Check sheet for the modelled part. Datum: model origin and axes. Units: mm. A direction names the side the tool comes from. Round coordinates to 2 decimals unless told otherwise and drop trailing zeros. Write each loop counter-clockwise with the first axis right and the second up, starting at its lowest first coordinate (ties: lowest second). Pieces come first, ordered by that corner, then holes. Notation, with made-up numbers: M 8.25,2.25 L 16.25,2.25 A19 ccw 16.25,11.25 Z; hole C 77.5,-1.5 d1. An arc over 180 degrees is marked long. Answer in a Markdown table with one row per item.
```python
from build123d import *

# Parameters (mm, degrees)
F1_DEPTH = 3.81


with BuildPart() as f1:
    # F0 (on Front) → F1 (new body)
    with BuildSketch(Plane.XZ):
        Polygon((24.534516, 6.574004), (0, 0), (25.4, 0), (19.930718, 2.623929), align=None)
        Polygon((-6.574004, 24.534516), (0, 0), (0, 25.4), (-2.623929, 19.930718), align=None)
        Polygon((-24.534516, -6.574004), (0, 0), (-25.4, 0), (-19.930718, -2.623929), align=None)
        Polygon((6.574004, -24.534516), (0, 0), (0, -25.4), (2.623929, -19.930718), align=None)
        Polygon((25.4, 0), (0, 0), (24.534516, -6.574004), (19.930718, -2.623929), align=None)
        Polygon((21.997045, 12.7), (0, 0), (24.534516, 6.574004), (18.572473, 7.69297), align=None)
        Polygon((17.960512, 17.960512), (0, 0), (21.997045, 12.7), (15.948544, 12.237748), align=None)
        Polygon((12.7, 21.997045), (0, 0), (17.960512, 17.960512), (12.237748, 15.948544), align=None)
        Polygon((6.574004, 24.534516), (0, 0), (12.7, 21.997045), (7.69297, 18.572473), align=None)
        Polygon((0, 25.4), (0, 0), (6.574004, 24.534516), (2.623929, 19.930718), align=None)
        Polygon((0, -25.4), (0, 0), (-6.574004, -24.534516), (-2.623929, -19.930718), align=None)
        Polygon((24.534516, -6.574004), (0, 0), (21.997045, -12.7), (18.572473, -7.69297), align=None)
        Polygon((21.997045, -12.7), (0, 0), (17.960512, -17.960512), (15.948544, -12.237748), align=None)
        Polygon((17.960512, -17.960512), (0, 0), (12.7, -21.997045), (12.237748, -15.948544), align=None)
        Polygon((12.7, -21.997045), (0, 0), (6.574004, -24.534516), (7.69297, -18.572473), align=None)
        Polygon((-6.574004, -24.534516), (0, 0), (-12.7, -21.997045), (-7.69297, -18.572473), align=None)
        Polygon((-12.7, -21.997045), (0, 0), (-17.960512, -17.960512), (-12.237748, -15.948544), align=None)
        Polygon((-17.960512, -17.960512), (0, 0), (-21.997045, -12.7), (-15.948544, -12.237748), align=None)
        Polygon((-21.997045, -12.7), (0, 0), (-24.534516, -6.574004), (-18.572473, -7.69297), align=None)
        Polygon((-25.4, 0), (0, 0), (-24.534516, 6.574004), (-19.930718, 2.623929), align=None)
        Polygon((-24.534516, 6.574004), (0, 0), (-21.997045, 12.7), (-18.572473, 7.69297), align=None)
        Polygon((-21.997045, 12.7), (0, 0), (-17.960512, 17.960512), (-15.948544, 12.237748), align=None)
        Polygon((-17.960512, 17.960512), (0, 0), (-12.7, 21.997045), (-12.237748, 15.948544), align=None)
        Polygon((-12.7, 21.997045), (0, 0), (-6.574004, 24.534516), (-7.69297, 18.572473), align=None)
    extrude(amount=F1_DEPTH)


solid = f1.part
```
1. Section check A-A, the plane z = -5. Record the cut outline in (x, y).
Found:
| item | result |
|---|---|
| outline | M -22.7,-3.81 L 22.7,-3.81 L 22.7,0 L -22.7,0 Z |
2. Draft check along Z on faces 5 (the face through (10.16, -1.88, -20.26)), 6 (the face through (-1.294, -1.878, 22.704)), 7 (the face through (-22.704, -1.878, -1.294)). Enter one of: +Z half, -Z half, draft (parallel to the pull), parting line (faces both ways), or undercut.
Found:
| item | result |
|---|---|
| face 5 | -Z half |
| face 6 | +Z half |
| face 7 | undercut |
3. Access from +Z, -Z, +X, -X, +Y, -Y to the whole of each face (thin tool, end or side, straight path). Record for faces 1 (the face through (22.63, -1.88, -1.33)), 2 (the face through (-20.26, -1.88, -10.16)), 3 (the face through (12.472, -1.878, -19.015)), 4 (the face through (-7.126, -1.878, 21.595)).
Found:
| item | result |
|---|---|
| face 1 | +X, +Y, -Y |
| face 2 | -X, +Y, -Y |
| face 3 | +Y, -Y |
| face 4 | +Z, +Y, -Y |
4. Section check B-B, the plane x = -11.5. Record the cut outline in (y, z).
Found:
| item | result |
|---|---|
| outline | M -3.81,-21.18 L 0,-21.18 L 0,21.18 L -3.81,21.18 Z |
5. Scan lines: L1, parallel to Z at x = -18, y = -3; L2, parallel to X at y = -3, z = -14.5; L3, parallel to X at y = -0.4, z = -4. Record each from-to range of solid material in increasing order.
Found:
| item | result |
|---|---|
| L1 | z = -12.39 to 12.39 |
| L2 | x = -16.74 to 16.74 |
| L3 | x = -21.53 to 21.53 |
6. Go/stop test with flat-tipped pins: pin 1 (1.5 mm diameter, centred on y = -1.5, z = -2.5, fed in from -X); pin 2 (2 mm diameter, centred on x = 8.5, y = -0.5, fed in from -Z). Record where each tip stops, or that it passes through.
Found:
| item | result |
|---|---|
| pin 1 | stops at x = -21.75 |
| pin 2 | stops at z = -19.81 |
